```python
from build123d import *

# Parameters (mm, degrees)
SKETCH1_W           = 24
SKETCH1_H           = 33
BOSS_EXTRUDE2_DEPTH = 3
SKETCH2_R           = 1.25
CUT_EXTRUDE2_DEPTH  = 3
SKETCH4_W           = 2.5
SKETCH4_H           = 33
BOSS_EXTRUDE3_DEPTH = 3
SKETCH5_W           = 2
SKETCH5_H           = 33
BOSS_EXTRUDE4_DEPTH = 15.5
SKETCH6_W           = 1
SKETCH6_H           = 33
CUT_EXTRUDE3_DEPTH  = 1


with BuildPart() as part:
    # Sketch1 → Boss-Extrude2 (new body)
    with BuildSketch(Plane(origin=(0, 0, 0), x_dir=(1, 0, 0), z_dir=(0, 1, 0))):
        Rectangle(SKETCH1_W, SKETCH1_H)
        with BuildLine():
            Line((10.5, 7), (10.5, 15))
            Line((10.5, 15), (-10.5, 15))
            Line((-10.5, 15), (-10.5, 7))
            ThreePointArc((-10.5, 7), (-7.5, 4), (-10.5, 1))
            Line((-10.5, 1), (-10.5, -15))
            Line((-10.5, -15), (10.5, -15))
            Line((10.5, -15), (10.5, 1))
            ThreePointArc((10.5, 1), (7.5, 4), (10.5, 7))
        make_face(mode=Mode.SUBTRACT)
    extrude(amount=BOSS_EXTRUDE2_DEPTH)

    # Sketch2 → Cut-Extrude2 (cut)
    with BuildSketch(Plane(origin=(0, 3, 0), x_dir=(1, 0, 0), z_dir=(0, 1, 0))):
        with Locations(Location((-10.5, 4, 0), (0, 0, 270))):
            Circle(SKETCH2_R)
        with Locations(Location((10.5, 4, 0), (0, 0, 270))):
            Circle(SKETCH2_R)
    extrude(amount=-CUT_EXTRUDE2_DEPTH, mode=Mode.SUBTRACT)

    # Sketch4 → Boss-Extrude3 (add)
    with BuildSketch(Plane(origin=(0, 3, 0), x_dir=(1, 0, 0), z_dir=(0, 1, 0))):
        with Locations((-13.25, 0)):
            Rectangle(SKETCH4_W, SKETCH4_H)
        with Locations((13.25, 0)):
            Rectangle(SKETCH4_W, SKETCH4_H)
    extrude(amount=-BOSS_EXTRUDE3_DEPTH)

    # Sketch5 → Boss-Extrude4 (add)
    with BuildSketch(Plane(origin=(0, 3, 0), x_dir=(1, 0, 0), z_dir=(0, 1, 0))):
        with Locations((-13.5, 0)):
            Rectangle(SKETCH5_W, SKETCH5_H)
        with Locations((13.5, 0)):
            Rectangle(SKETCH5_W, SKETCH5_H)
    extrude(amount=BOSS_EXTRUDE4_DEPTH)

    # Sketch6 → Cut-Extrude3 (cut)
    with BuildSketch(Plane(origin=(0, 18.5, 0), x_dir=(1, 0, 0), z_dir=(0, 1, 0))):
        with Locations((13.5, 0)):
            Rectangle(SKETCH6_W, SKETCH6_H)
        with Locations((-13.5, 0)):
            Rectangle(SKETCH6_W, SKETCH6_H)
    extrude(amount=-CUT_EXTRUDE3_DEPTH, mode=Mode.SUBTRACT)


solid = part.part
```
Geometry: final body of the model. Coordinates: model frame, mm. A direction names the side the tool comes from. Round coordinates to 2 decimals unless told otherwise and drop trailing zeros. Write each loop counter-clockwise with the first axis right and the second up, starting at its lowest first coordinate (ties: lowest second). Pieces come first, ordered by that corner, then holes. Notation, with made-up numbers: M -9.75,26 L 25.25,26 A24 cw 25.25,64 Z; hole C 47,20 d6. An arc over 180 degrees is marked long. Answer in a Markdown table with one row per item. Add a question column.
(1) Draft query along X for faces 1 (the face through (7.5, 1.5, -3.9)), 2 (the face through (14.5, 9, 0)), 3 (the face through (-14.5, 9, 0)). Return one class per face: pulls with the +X half, pulls with the -X half, needs draft (parallel to the pull), parting line crosses it, or undercut.
(2) Cut plane A-A, the plane z = 14. Return the cut outline in (x, y), then the cut area to 3 significant figures.
(3) Cut plane C-C, the plane x = 8. Return the cut outline in (y, z), then the cut area to 3 significant figures.
(4) Reachability of faces 4 (the face through (10.5, 1, -11)), 5 (the face through (0, 1, -16.5)), 6 (the face through (-12.5, 11, 0)) from +Z, -Z, +X, -X, +Y, -Y: full face, straight path, thin tool, end or side. Return the list, or none.
(5) Cut plane D-D, the plane z = -4. Return the cut outline in (x, y), then the cut area to 3 significant figures.
(6) Ray query, L1, parallel to X at y = 1.05, z = -4; L2, parallel to X at y = 15, z = 13.5; L3, parallel to X at y = 1.75, z = 10. Return the intervals inside material, ascending.
(7) Cut plane B-B, the plane y = 13.5. Return the cut outline in (x, z), then the cut area to 3 significant figures.
(8) Contact query for flat-ended pins moving along their axis: pin 1 (12.5 mm diameter, centred on x = -5, z = 2, fed in from +Y); pin 2 (0.5 mm diameter, centred on x = 13.5, z = -7, fed in from +Y); pin 3 (2 mm diameter, centred on x = 10.5, z = -4, fed in from +Y). Output: stop coordinate, or through.
Established:
| question | item | result |
|---|---|---|
| 1 | face 1 | undercut |
| 1 | face 2 | pulls with the +X half |
| 1 | face 3 | pulls with the -X half |
| 2 | outline | M -14.5,0 L -10.5,0 L -10.5,3 L -12.5,3 L -12.5,18.5 L -13,18.5 L -13,17.5 L -14,17.5 L -14,18.5 L -14.5,18.5 Z; M 10.5,0 L 14.5,0 L 14.5,18.5 L 14,18.5 L 14,17.5 L 13,17.5 L 13,18.5 L 12.5,18.5 L 12.5,3 L 10.5,3 Z |
| 2 | area | 84.0 mm² |
| 3 | outline | M 0,-16.5 L 3,-16.5 L 3,-15 L 0,-15 Z; M 0,-5.66 L 3,-5.66 L 3,-2.34 L 0,-2.34 Z; M 0,15 L 3,15 L 3,16.5 L 0,16.5 Z |
| 3 | area | 18.9 mm² |
| 4 | face 4 | +Y, -Y |
| 4 | face 5 | -Z, +X, -X, +Y, -Y |
| 4 | face 6 | +Z, -Z, +Y |
| 5 | outline | M -14.5,0 L -11.75,0 L -11.75,3 L -12.5,3 L -12.5,18.5 L -13,18.5 L -13,17.5 L -14,17.5 L -14,18.5 L -14.5,18.5 Z; M -9.25,0 L -7.5,0 L -7.5,3 L -9.25,3 Z; M 7.5,0 L 9.25,0 L 9.25,3 L 7.5,3 Z; M 11.75,0 L 14.5,0 L 14.5,18.5 L 14,18.5 L 14,17.5 L 13,17.5 L 13,18.5 L 12.5,18.5 L 12.5,3 L 11.75,3 Z |
| 5 | area | 87.0 mm² |
| 6 | L1 | -14.5 to -11.75, -9.25 to -7.5, 7.5 to 9.25, 11.75 to 14.5 |
| 6 | L2 | -14.5 to -12.5, 12.5 to 14.5 |
| 6 | L3 | -14.5 to -10.5, 10.5 to 14.5 |
| 7 | outline | M -14.5,-16.5 L -12.5,-16.5 L -12.5,16.5 L -14.5,16.5 Z; M 12.5,-16.5 L 14.5,-16.5 L 14.5,16.5 L 12.5,16.5 Z |
| 7 | area | 132 mm² |
| 8 | pin 1 | y = 3 |
| 8 | pin 2 | y = 17.5 |
| 8 | pin 3 | through |
